For this review, take the finished solid that the model builds, in its own axes (mm). Face numbers are marked on the shaded views. A direction names the side the tool comes from. Coordinates: 2 decimals unless noted, no trailing zeros. Loops run counter-clockwise (first coordinate to the right, second up) from the corner with the lowest first, then second, coordinate; pieces in that order, holes last. Notation, with made-up numbers: (-35, 13) -> (-3, 13) arc R33 ccw to (-3, 47) -> close; hole circle Ø4 at (54, 25). An arc over 180 degrees is marked (long way). Answer in a Markdown table with one row per item.
from build123d import *

# Parameters (mm, degrees)
F0_W      = 76.2
F0_H      = 76.2
F1_DEPTH  = 76.2
F2_W      = 57.15
F2_H      = 57.15
F3_DEPTH  = 57.15
F4_SIZE   = 6.35
F5_SIZE   = 6.35
F6_R      = 5.08
F7_R      = 12.7
F8_DEPTH  = 19.05
F9_R      = 12.7
F10_DEPTH = 19.05
F11_R     = 12.7
F12_DEPTH = 19.05


with BuildPart() as f1:
    # F0 (on Front) → F1 (new body)
    with BuildSketch(Plane.XZ):
        Rectangle(F0_W, F0_H)
    extrude(amount=F1_DEPTH)

    # F2 (on face) → F3 (cut)
    with BuildSketch(Plane.XZ.offset(76.2)):
        with Locations((9.525, 9.525)):
            Rectangle(F2_W, F2_H)
    extrude(amount=-F3_DEPTH, mode=Mode.SUBTRACT)

    # F4
    f4_edges = [f1.edges().sort_by_distance(p)[0] for p in [
        (-28.575, -76.2, 38.1),
    ]]
    chamfer(f4_edges, length=F4_SIZE)

    # F5
    f5_edges = [f1.edges().sort_by_distance(p)[0] for p in [
        (38.1, -9.525, 38.1),
    ]]
    chamfer(f5_edges, length=F5_SIZE)

    # F6
    f6_edges = [f1.edges().sort_by_distance(p)[0] for p in [
        (-19.05, -19.05, 9.525),
    ]]
    fillet(f6_edges, radius=F6_R)

    # F7 (on face) → F8 (cut)
    with BuildSketch(Plane.YZ.offset(-19.05)):
        with Locations((-47.625, 9.525)):
            Circle(F7_R)
    extrude(amount=-F8_DEPTH, mode=Mode.SUBTRACT)

    # F9 (on face) → F10 (cut)
    with BuildSketch(Plane.XZ.offset(19.05)):
        with Locations((9.525, 9.525)):
            Circle(F9_R)
    extrude(amount=-F10_DEPTH, mode=Mode.SUBTRACT)

    # F11 (on face) → F12 (cut)
    with BuildSketch(Plane.XY.offset(-19.05)):
        with Locations((9.525, -47.625)):
            Circle(F11_R)
    extrude(amount=-F12_DEPTH, mode=Mode.SUBTRACT)


solid = f1.part
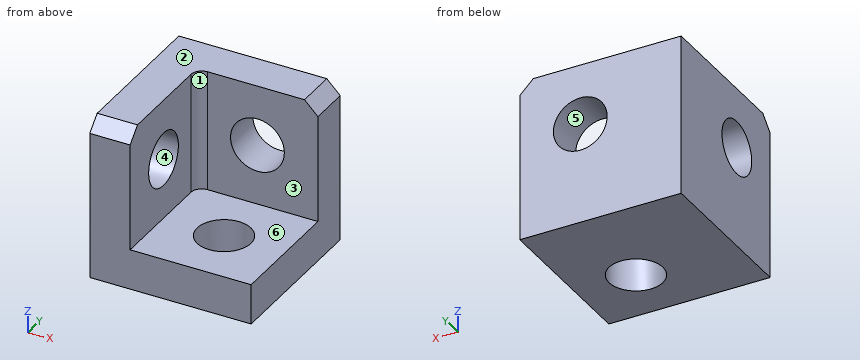
Item 1: Take a section at A-A, the plane x = 4. State the section outline as (y, z) points, and give its area (3 significant figures).
Worked answers:
| item | result |
|---|---|
| outline | (-76.2, -38.1) -> (-59.06, -38.1) -> (-59.06, -19.05) -> (-76.2, -19.05) -> close; (-36.19, -38.1) -> (0, -38.1) -> (0, -1.91) -> (-19.05, -1.91) -> (-19.05, -19.05) -> (-36.19, -19.05) -> close; (-19.05, 20.96) -> (0, 20.96) -> (0, 38.1) -> (-19.05, 38.1) -> close |
| area | 1,670 mm² |
Item 2: For the marked faces 1 and 2, list the 3-axis set-ups (+Z, -Z, +X, -X, +Y, -Y) from which the entire face can be reached by the end or side of a thin tool; tool diameter is ignored.
Worked answers:
| item | result |
|---|---|
| face 1 | +Z, +X, -Y |
| face 2 | +Z, +X, -X, +Y, -Y |
Item 3: The part is to be moulded in two halves that separate along Z. For the marked faces 3, 4, 5 and 6, say which applies: +Z half, -Z half, draft (parallel to the pull), parting line (faces both ways), or undercut.
Worked answers:
| item | result |
|---|---|
| face 3 | draft |
| face 4 | undercut |
| face 5 | undercut |
| face 6 | +Z half |
Item 4: For L1, parallel to X at y = -58, z = -15.5; L2, parallel to Y at x = -4, z = 1, list the stretches that pass through material, from the lowest coordinate up.
Worked answers:
| item | result |
|---|---|
| L1 | -38.1 to -19.05 |
| L2 | -19.05 to 0 |
Item 5: Take a section at B-B, the plane z = 33.5. State the section outline as (x, y) points.
Worked answers:
| item | result |
|---|---|
| outline | (-38.1, -74.45) -> (-19.05, -74.45) -> (-19.05, -24.13) arc R5.08 cw to (-13.97, -19.05) -> (36.35, -19.05) -> (36.35, 0) -> (-38.1, 0) -> close |
Item 6: Take a section at D-D, the plane z = 7.5. State the section outline as (x, y) points, and give its area (3 significant figures).
Worked answers:
| item | result |
|---|---|
| outline | (-38.1, -76.2) -> (-19.05, -76.2) -> (-19.05, -60.16) -> (-38.1, -60.16) -> close; (-38.1, -35.09) -> (-19.05, -35.09) -> (-19.05, -24.13) arc R5.08 cw to (-13.97, -19.05) -> (-3.01, -19.05) -> (-3.01, 0) -> (-38.1, 0) -> close; (22.06, -19.05) -> (38.1, -19.05) -> (38.1, 0) -> (22.06, 0) -> close |
| area | 1,590 mm² |
Item 7: Insertion check: pin 1 (10 mm diameter, centred on x = 26, z = -9.5, fed in from -Y); pin 2 (2 mm diameter, centred on y = -42.5, z = -8.5, fed in from +X). Each pin has a flat end and moves straight along its axis. Give the tip position at first contact, or say it passes through.
Worked answers:
| item | result |
|---|---|
| pin 1 | y = -19.05 |
| pin 2 | x = -19.05 |
Item 8: Take a section at C-C, the plane y = -41.5. State the section outline as (x, z) points.
Worked answers:
| item | result |
|---|---|
| outline | (-38.1, -38.1) -> (-1.6, -38.1) -> (-1.6, -19.05) -> (-19.05, -19.05) -> (-19.05, -1.6) -> (-38.1, -1.6) -> close; (-38.1, 20.65) -> (-19.05, 20.65) -> (-19.05, 38.1) -> (-38.1, 38.1) -> close; (20.65, -38.1) -> (38.1, -38.1) -> (38.1, -19.05) -> (20.65, -19.05) -> close |
